```python
from build123d import *

# Parameters (mm, degrees)
SKETCH1_W                        = 117.475
SKETCH1_H                        = 35.56
EXTRUDE1_DEPTH                   = 119.38
SKETCH2_W                        = 41.402
SKETCH2_H                        = 20.828
EXTRUDE2_DEPTH                   = 15.494
F_25_64_0_39063_DIAMETER_HOLE1_D = 9.922002
SHELL1_T                         = -2.54


with BuildPart() as part:
    # Sketch1 → Extrude1 (new body)
    with BuildSketch(Plane.XY):
        Rectangle(SKETCH1_W, SKETCH1_H)
    extrude(amount=EXTRUDE1_DEPTH)

    # Sketch2 → Extrude2 (add)
    with BuildSketch(Plane(origin=(0, 0, 0), x_dir=(-1, 0, 0), z_dir=(0, 0, -1))):
        Rectangle(SKETCH2_W, SKETCH2_H)
    extrude(amount=EXTRUDE2_DEPTH)

    # 25/64 (0.39063) Diameter Hole1 (through all)
    with Locations(Plane(origin=(-51.1175, -17.78, 43.688), x_dir=(0, 0, -1), z_dir=(0, -1, 0))):
        with Locations((0, 0), (0, 102.235)):
            Hole(F_25_64_0_39063_DIAMETER_HOLE1_D / 2)

    # Shell1
    shell1_openings = [part.faces().sort_by_distance(p)[0] for p in [
        (0, 0, 119.38),
    ]]
    offset(amount=SHELL1_T, openings=shell1_openings, kind=Kind.INTERSECTION)


solid = part.part
```
Geometry: final body of the model. Coordinates: model frame, mm. A direction names the side the tool comes from. Coordinates: 2 decimals unless noted, no trailing zeros. Order: outer loops, then holes, each group sorted by start corner. A loop starts at its lowest first (then second) coordinate and runs counter-clockwise, first axis right, second up. Notation, with made-up numbers: (81, -24) -> (124, -24) arc R28 ccw to (124, 2) -> close; hole circle Ø3 at (60.5, 14). An arc over 180 degrees is marked (long way). Write each question's results on one line, items separated by ' | '. Start each with the question number.
1) Mould query, pull axis Y, two halves, no side actions, for faces 1 (the flat face through (0, 10.414, -8)), 2 (the flat face through (-20.701, 0, -8)), 3 (the flat face through (-1, 15.24, 60)), 4 (the flat face through (0, -10.414, -8)). Classes: released by +Y, released by -Y, zero draft, split by the parting line, or undercut.
2) Cut plane B-B, the plane z = -1.5. Output: boundary loops of the cut face in (x, y).
3) Cut plane C-C, the plane y = 5. Output: boundary loops of the cut face in (x, z), and give its area (3 significant figures).
4) Material intervals for line 1 along Z through (x, y) = (51, 9.5); line 2 along X through (y, z) = (4.5, 44); line 3 along X through (y, z) = (-15, 21.5), sorted ascending.
5) Set-up query: faces 5 (the flat face through (-1, 10, 2.54)), 6 (the flat face through (56.198, 0, 84)), 7 (the flat face through (20.701, 0, -8)). Return all of +Z, -Z, +X, -X, +Y, -Y with unobstructed straight access to the full face (end or side cutting, diameter ignored); none if empty.
6) Cut plane D-D, the plane x = -3.5. Output: boundary loops of the cut face in (y, z), and give its area (3 significant figures).
7) First-contact query: pin 1 (17 mm diameter, centred on y = -4, z = -4, fed in from -X); pin 2 (4.5 mm diameter, centred on x = -7, z = -5.5, fed in from -Y); pin 3 (4.5 mm diameter, centred on x = -4, y = -2, fed in from +Z); pin 4 (4.5 mm diameter, centred on y = 3.5, z = -8.5, fed in from +X). Flat tips, straight axial feed; report the tip coordinate or a pass-through.
8) Cut plane A-A, the plane x = -49. Output: boundary loops of the cut face in (y, z).
Checks:
1) face 1: released by +Y | face 2: zero draft | face 3: undercut | face 4: released by -Y
2) outline: (-20.7, -10.41) -> (20.7, -10.41) -> (20.7, 10.41) -> (-20.7, 10.41) -> close; hole (-18.16, -7.87) -> (18.16, -7.87) -> (18.16, 7.87) -> (-18.16, 7.87) -> close
3) outline: (-58.74, 0) -> (-20.7, 0) -> (-20.7, -15.49) -> (20.7, -15.49) -> (20.7, 0) -> (58.74, 0) -> (58.74, 119.38) -> (56.2, 119.38) -> (56.2, 49.21) arc R7.5 ccw (long way) to (56.2, 38.17) -> (56.2, 2.54) -> (18.16, 2.54) -> (18.16, -12.95) -> (-18.16, -12.95) -> (-18.16, 2.54) -> (-56.2, 2.54) -> (-56.2, 38.17) arc R7.5 ccw (long way) to (-56.2, 49.21) -> (-56.2, 119.38) -> (-58.74, 119.38) -> close; hole circle Ø9.92 at (-51.12, 43.69); hole circle Ø9.92 at (51.12, 43.69) | area: 1,130 mm^2
4) line 1: 0 to 2.54, 36.19 to 38.73, 48.65 to 51.19 | line 2: -58.74 to -56.07, -46.17 to -43.62, 43.62 to 46.17, 56.07 to 58.74 | line 3: -58.74 to -56.2, 56.2 to 58.74
5) face 5: none | face 6: +Z | face 7: -Z, +X, +Y, -Y
6) outline: (-17.78, 0) -> (-10.41, 0) -> (-10.41, -15.49) -> (10.41, -15.49) -> (10.41, 0) -> (17.78, 0) -> (17.78, 119.38) -> (15.24, 119.38) -> (15.24, 2.54) -> (7.87, 2.54) -> (7.87, -12.95) -> (-7.87, -12.95) -> (-7.87, 2.54) -> (-15.24, 2.54) -> (-15.24, 119.38) -> (-17.78, 119.38) -> close | area: 763 mm^2
7) pin 1: x = -58.74 | pin 2: y = -10.41 | pin 3: z = -12.95 | pin 4: x = 20.7
8) outline: (-17.78, 0) -> (17.78, 0) -> (17.78, 39.2) -> (-17.78, 39.2) -> close; (-17.78, 48.17) -> (17.78, 48.17) -> (17.78, 119.38) -> (15.24, 119.38) -> (15.24, 50.88) -> (-15.24, 50.88) -> (-15.24, 119.38) -> (-17.78, 119.38) -> close; hole (-15.24, 2.54) -> (15.24, 2.54) -> (15.24, 36.49) -> (-15.24, 36.49) -> close
